Input: part model. Units: mm. Frame: model coordinates. Face numbers are marked on the shaded views. A direction names the side the tool comes from. Round coordinates to 2 decimals unless told otherwise and drop trailing zeros. Write each loop counter-clockwise with the first axis right and the second up, starting at its lowest first coordinate (ties: lowest second). Pieces come first, ordered by that corner, then holes. Notation, with made-up numbers: (30.25, 51) -> (81.25, 51) arc R25 cw to (81.25, 72) -> close; hole circle Ø4 at (1, -15.5). An arc over 180 degrees is marked (long way). Write item = value, one per line.
```python
from build123d import *

# Parameters (mm, degrees)
BOSS_EXTRUDE1_DEPTH = 20
SKETCH6_W           = 10
SKETCH6_H           = 10
CUT_EXTRUDE2_DEPTH  = 5
SKETCH7_W           = 10
SKETCH7_H           = 10
CUT_EXTRUDE3_DEPTH  = 5
FILLET1_R           = 2
FILLET2_R           = 2
CUT_EXTRUDE4_DEPTH  = 30
SKETCH9_W           = 43
SKETCH9_H           = 15
CUT_EXTRUDE5_DEPTH  = 25


with BuildPart() as part:
    # Sketch1 → Boss-Extrude1 (new body)
    with BuildSketch(Plane.XY):
        Polygon((-27.5, 32.5), (27.5, 32.5), (27.5, -2.5), (21.5, -2.5), (21.5, -32.5), (-21.5, -32.5), (-21.5, -2.5), (-27.5, -2.5), align=None)
    extrude(amount=BOSS_EXTRUDE1_DEPTH)

    # Sketch6 → Cut-Extrude2 (cut)
    with BuildSketch(Plane(origin=(0, 32.5, 0), x_dir=(1, 0, 0), z_dir=(0, 1, 0))):
        with Locations((-17.5, -10)):
            Rectangle(SKETCH6_W, SKETCH6_H)
        with Locations((17.5, -10)):
            Rectangle(SKETCH6_W, SKETCH6_H)
    extrude(amount=-CUT_EXTRUDE2_DEPTH, mode=Mode.SUBTRACT)

    # Sketch7 → Cut-Extrude3 (cut)
    with BuildSketch(Plane.XZ.offset(32.5)):
        with Locations((-14, 7.5)):
            Rectangle(SKETCH7_W, SKETCH7_H)
        with Locations((14, 7.5)):
            Rectangle(SKETCH7_W, SKETCH7_H)
    extrude(amount=-CUT_EXTRUDE3_DEPTH, mode=Mode.SUBTRACT)

    # Fillet1
    fillet1_edges = [part.edges().sort_by_distance(p)[0] for p in [
        (-21.5, -17.5, 0),
        (-27.5, 15, 0),
        (-27.5, 32.5, 10),
        (27.5, 32.5, 10),
        (27.5, -2.5, 10),
        (-21.5, -32.5, 10),
        (-27.5, -2.5, 10),
        (0, -32.5, 20),
        (21.5, -17.5, 20),
        (27.5, 15, 20),
        (0, 32.5, 20),
        (-27.5, 15, 20),
        (0, 32.5, 0),
        (27.5, 15, 0),
        (21.5, -17.5, 0),
    ]]
    fillet(fillet1_edges, radius=FILLET1_R)

    # Fillet2
    # the kernel refuses this fillet: 2 mm, written as the material it takes off along each edge
    with BuildSketch(Plane(origin=(-19.5, -30.5, 2), x_dir=(0, 0, -1), z_dir=(0, -1, 0))) as fillet2_piece_1_section:
        Polygon((0, 0), (FILLET2_R, 0), (FILLET2_R, -FILLET2_R), (0, -FILLET2_R), align=None)
    fillet2_piece_1 = extrude(amount=FILLET2_R, mode=Mode.PRIVATE)
    fillet2_piece_1 = fillet2_piece_1 - Plane(origin=(-19.5, -30.5, 2), x_dir=(0.7071067811865475, 0, 0.7071067811865475), z_dir=(0, -1, 0)) * Sphere(FILLET2_R, mode=Mode.PRIVATE)
    add(fillet2_piece_1, mode=Mode.SUBTRACT)
    with BuildSketch(Plane(origin=(19.5, -30.5, 18), x_dir=(1, 0, 0), z_dir=(0, -1, 0))) as fillet2_piece_2_section:
        Polygon((0, 0), (FILLET2_R, 0), (FILLET2_R, FILLET2_R), (0, FILLET2_R), align=None)
    fillet2_piece_2 = extrude(amount=FILLET2_R, mode=Mode.PRIVATE)
    fillet2_piece_2 = fillet2_piece_2 - Plane(origin=(19.5, -30.5, 18), x_dir=(-0.7071067811865475, 0, -0.7071067811865475), z_dir=(0, -1, 0)) * Sphere(FILLET2_R, mode=Mode.PRIVATE)
    add(fillet2_piece_2, mode=Mode.SUBTRACT)
    with BuildSketch(Plane(origin=(21.5, -32.5, 2), x_dir=(-1, 0, 0), z_dir=(0, 0, 1))) as fillet2_piece_3:
        with BuildLine():
            CenterArc((FILLET2_R, -FILLET2_R), FILLET2_R, 90, 90)
            Line((0, -FILLET2_R), (0, 0))
            Line((0, 0), (FILLET2_R, 0))
        make_face()
    extrude(amount=16, mode=Mode.SUBTRACT)
    with BuildSketch(Plane(origin=(19.5, -32.5, 0), x_dir=(0, 0, 1), z_dir=(-1, 0, 0))) as fillet2_piece_4:
        with BuildLine():
            CenterArc((FILLET2_R, FILLET2_R), FILLET2_R, 180, 90)
            Line((0, FILLET2_R), (0, 0))
            Line((0, 0), (FILLET2_R, 0))
        make_face()
    extrude(amount=39, mode=Mode.SUBTRACT)
    with BuildSketch(Plane(origin=(19.5, -32.5, 2), x_dir=(0, 0, -1), z_dir=(-1, 0, 0))) as fillet2_piece_5:
        with BuildLine():
            CenterArc((2 - FILLET2_R, -FILLET2_R), FILLET2_R, 360, 90)
            Line((2, -FILLET2_R), (2, 0))
            Line((2, 0), (2 - FILLET2_R, 0))
        make_face()
    revolve(axis=Axis((19.5, -32.5, 2), (0, -1, 0)), revolution_arc=90, mode=Mode.SUBTRACT)

    # Sketch8 → Cut-Extrude4 (cut)
    with BuildSketch(Plane(origin=(0, -2.5, 0), x_dir=(-1, 0, 0), z_dir=(0, -1, 0))):
        Polygon((-23.544279595, 2.278765761), (24.281911255, 2.554989635), (24.437245142, -24.339963353), (-23.544279595, -24.339963353), align=None)
    extrude(amount=CUT_EXTRUDE4_DEPTH, mode=Mode.SUBTRACT)

    # Sketch9 → Cut-Extrude5 (cut)
    with BuildSketch(Plane.XZ.offset(2.5)):
        with Locations((0, 10)):
            Rectangle(SKETCH9_W, SKETCH9_H)
    extrude(amount=-CUT_EXTRUDE5_DEPTH, mode=Mode.SUBTRACT)


solid = part.part
```
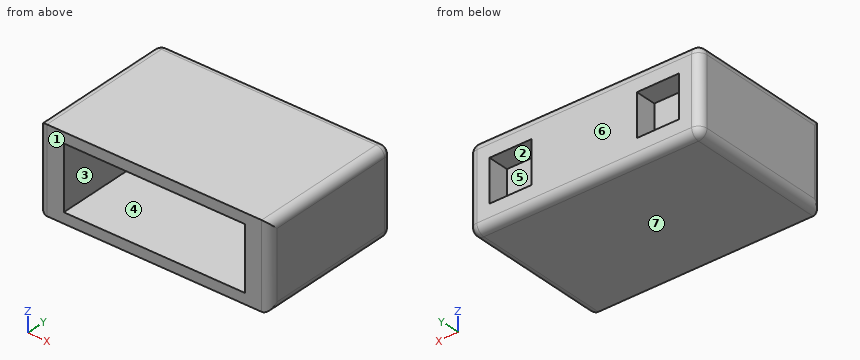
1) Cut plane B-B (y = 28.5). Return the cut outline in (x, z).
Solutions:
outline = (-27.5, 2) arc R2 ccw to (-25.5, 0) -> (25.5, 0) arc R2 ccw to (27.5, 2) -> (27.5, 18) arc R2 ccw to (25.5, 20) -> (-25.5, 20) arc R2 ccw to (-27.5, 18) -> close; hole (-22.5, 5) -> (-12.5, 5) -> (-12.5, 15) -> (-22.5, 15) -> close; hole (12.5, 5) -> (22.5, 5) -> (22.5, 15) -> (12.5, 15) -> close
2) Cut plane D-D (x = 17). Return the cut outline in (y, z), and give its area (3 significant figures).
Solutions:
outline = (-2.5, 0) -> (30.5, 0) arc R2 ccw to (32.5, 2) -> (32.5, 5) -> (27.5, 5) -> (27.5, 15) -> (32.5, 15) -> (32.5, 18) arc R2 ccw to (30.5, 20) -> (-2.5, 20) -> (-2.5, 17.5) -> (22.5, 17.5) -> (22.5, 2.5) -> (-2.5, 2.5) -> close
area = 273 mm^2
3) Line query: L1, parallel to X at y = 29, z = 6.5; L2, parallel to Z at x = -18.5, y = 9.5; L3, parallel to X at y = 18, z = 11.75. Output: solid intervals per line, ascending. Write a range as from..to.
Solutions:
L1 = -27.5..-22.5, -12.5..12.5, 22.5..27.5
L2 = 0..2.5, 17.5..20
L3 = -27.5..-21.5, 21.5..27.5
4) Cut plane C-C (z = 9.25). Return the cut outline in (x, y).
Solutions:
outline = (-27.5, -0.5) arc R2 ccw to (-25.5, -2.5) -> (-21.5, -2.5) -> (-21.5, 22.5) -> (21.5, 22.5) -> (21.5, -2.5) -> (25.5, -2.5) arc R2 ccw to (27.5, -0.5) -> (27.5, 30.5) arc R2 ccw to (25.5, 32.5) -> (22.5, 32.5) -> (22.5, 27.5) -> (12.5, 27.5) -> (12.5, 32.5) -> (-12.5, 32.5) -> (-12.5, 27.5) -> (-22.5, 27.5) -> (-22.5, 32.5) -> (-25.5, 32.5) arc R2 ccw to (-27.5, 30.5) -> close
5) Access query for the marked faces 1, 2 and 3. Directions: +Z, -Z, +X, -X, +Y, -Y. A direction counts if a zero-diameter tool reaches every point of the face in a straight line with its end or side. Return the directions, or none.
Solutions:
face_1 = +Z, -Z, +X, -X, -Y
face_2 = +Y
face_3 = -Y
6) Cut plane A-A (y = 20). Return the cut outline in (x, z), and give its area (3 significant figures).
Solutions:
outline = (-27.5, 2) arc R2 ccw to (-25.5, 0) -> (25.5, 0) arc R2 ccw to (27.5, 2) -> (27.5, 18) arc R2 ccw to (25.5, 20) -> (-25.5, 20) arc R2 ccw to (-27.5, 18) -> close; hole (-21.5, 2.5) -> (21.5, 2.5) -> (21.5, 17.5) -> (-21.5, 17.5) -> close
area = 452 mm^2
7) Draft query along Z for the marked faces 4, 5, 6 and 7. Return one class per face: +Z half, -Z half, draft (parallel to the pull), parting line (faces both ways), or undercut.
Solutions:
face_4 = undercut
face_5 = undercut
face_6 = draft
face_7 = -Z half
8) First-contact query: P1, Ø7.5, axis at x = -4, z = 12, coming from the -Y side; P2, Ø4, axis at y = 31, z = 7.5, coming from the +X side; P3, Ø3, axis at x = -18.5, z = 11.5, coming from the +Y side. Flat tips, straight axial feed; report the tip coordinate or a pass-through.
Solutions:
P1 = 22.5
P2 = 27.5
P3 = 27.5
